Could you check a few things on this model? Use its own coordinates, in mm. Face numbers are marked on the shaded views. A direction names the side the tool comes from. Coordinates: 2 decimals unless noted, no trailing zeros. Write each loop counter-clockwise with the first axis right and the second up, starting at its lowest first coordinate (ties: lowest second). Pieces come first, ordered by that corner, then holes. Notation, with made-up numbers: (9, -24) - (19, -24) arc R23 ccw to (19, -9) - close; hole circle Ø10 at (-14, 58.5). An arc over 180 degrees is marked (long way). Answer as a JSON object with one key per item and string values. Group by question number.
1) On a 3-axis mill with a long thin cutter (end or side, diameter ignored), from which of +Z, -Z, +X, -X, +Y, -Y can I reach the whole of each face in a straight line? I mean the marked faces 1 and 2. Say none if no direction works.
2) If we section it at D-D (x = -20): Write out the boundary of the cut face in (y, z).
3) We'd pull the mould along Z, two halves only. Please class the marked faces 3 and 4: released by +Z, released by -Z, zero draft, split by the parting line, or undercut.
4) Will these pins go through, and if not, where does the flat tip stop? pin 1 Ø1 at (x, z) = (1.5, 21.5) entering from +Y; pin 2 Ø2 at (x, y) = (28, 6) entering from -Z; pin 3 Ø2 at (x, y) = (-30.5, 7) entering from +Z.
5) If we section it at B-B (z = 48): Write out the boundary of the cut face in (x, y).
6) Please list where these lines run through material, in increasing order: line 1 along Z through (x, y) = (-27.5, 5.5); line 2 along X through (y, z) = (20, 34.5); line 3 along Y through (x, z) = (-30, 4).
7) If we section it at C-C (y = 6.5): State how many separate pieces and enclosed holes the cut face has, plus the area to 3 significant figures.
8) If we section it at A-A (x = -30): Write out the boundary of the cut face in (y, z).
```python
from build123d import *

# Parameters (mm, degrees)
SKETCH1_W                                           = 75
SKETCH1_H                                           = 5
SKETCH1_W_2                                         = 5
SKETCH1_H_2                                         = 40
BOSS_EXTRUDE1_DEPTH                                 = 90
SKETCH2_R                                           = 2.1
CUT_EXTRUDE1_DEPTH                                  = 122.680935236
SKETCH4_W                                           = 4
SKETCH4_H                                           = 90
BOSS_EXTRUDE2_DEPTH                                 = 40
SKETCH6_W                                           = 7
SKETCH6_H                                           = 4
BOSS_EXTRUDE4_DEPTH                                 = 8
SKETCH7_R                                           = 1.6
CUT_EXTRUDE3_DEPTH                                  = 106.386194542
CUT_EXTRUDE4_REACH                                  = 126.624
LPATTERN1_COUNT                                     = 5
LPATTERN1_PITCH                                     = 12
SKETCH9_R                                           = 1.5
CUT_EXTRUDE5_DEPTH                                  = 104.834002138
CSK_FOR_M4_COUNTERSUNK_FLAT_HEAD_SCREW1_D           = 4
CSK_FOR_M4_COUNTERSUNK_FLAT_HEAD_SCREW1_CSINK_D     = 7.5
CSK_FOR_M4_COUNTERSUNK_FLAT_HEAD_SCREW1_CSINK_ANGLE = 90


with BuildPart() as part:
    # Sketch1 → Boss-Extrude1 (new body)
    with BuildSketch(Plane.XY):
        Rectangle(SKETCH1_W, SKETCH1_H)
        with Locations((35, 22.5)):
            Rectangle(SKETCH1_W_2, SKETCH1_H_2)
    extrude(amount=BOSS_EXTRUDE1_DEPTH)

    # Sketch2 → Cut-Extrude1 (cut, through all)
    with BuildSketch(Plane.ZY.offset(-32.5)):
        with Locations((20, 19.5)):
            Circle(SKETCH2_R)
        with Locations((70, 19.5)):
            Circle(SKETCH2_R)
    extrude(amount=-CUT_EXTRUDE1_DEPTH, mode=Mode.SUBTRACT)

    # Sketch4 → Boss-Extrude2 (add)
    with BuildSketch(Plane(origin=(0, 2.5, 0), x_dir=(1, 0, 0), z_dir=(0, 1, 0))):
        with Locations((-35.5, -45)):
            Rectangle(SKETCH4_W, SKETCH4_H)
    extrude(amount=BOSS_EXTRUDE2_DEPTH)

    # Sketch6 → Boss-Extrude4 (add)
    with BuildSketch(Plane(origin=(0, 2.5, 0), x_dir=(1, 0, 0), z_dir=(0, 1, 0))):
        with Locations((-30, -5)):
            Rectangle(SKETCH6_W, SKETCH6_H)
        with Locations((29, -5)):
            Rectangle(SKETCH6_W, SKETCH6_H)
        with Locations((29, -85)):
            Rectangle(SKETCH6_W, SKETCH6_H)
        with Locations((-30, -85)):
            Rectangle(SKETCH6_W, SKETCH6_H)
    extrude(amount=BOSS_EXTRUDE4_DEPTH)

    # Sketch7 → Cut-Extrude3 (cut, through all)
    with BuildSketch(Plane(origin=(0, 2.5, 0), x_dir=(1, 0, 0), z_dir=(0, 1, 0))):
        with Locations(Location((24.5, -68, 0), (0, 0, 180))):
            Circle(SKETCH7_R)
        with Locations(Location((-8.5, -17, 0), (0, 0, 180))):
            Circle(SKETCH7_R)
    extrude(amount=-CUT_EXTRUDE3_DEPTH, mode=Mode.SUBTRACT)

    # Sketch8 → Cut-Extrude4 (cut, up to next)
    with BuildSketch(Plane.ZY.offset(37.5), mode=Mode.PRIVATE) as cut_extrude4_sk1:
        with BuildLine():
            Line((32.061260163, 34.989949494), (32.202681519, 34.848528137))
            ThreePointArc((32.202681519, 34.848528137), (32.612732026, 33.858578644), (32.202681519, 32.86862915))
            Line((32.202681519, 32.86862915), (10.989949494, 11.655897124))
            ThreePointArc((10.989949494, 11.655897124), (10, 11.245846618), (9.010050506, 11.655897124))
            Line((9.010050506, 11.655897124), (8.86862915, 11.797318481))
            ThreePointArc((8.86862915, 11.797318481), (8.458578644, 12.787267974), (8.86862915, 13.777217468))
            Line((8.86862915, 13.777217468), (30.081361176, 34.989949494))
            ThreePointArc((30.081361176, 34.989949494), (31.07131067, 35.4), (32.061260163, 34.989949494))
        make_face()
    cut_extrude4_tool1 = extrude(cut_extrude4_sk1.sketch, amount=-CUT_EXTRUDE4_REACH, mode=Mode.PRIVATE) & part.part
    cut_extrude4 = cut_extrude4_tool1.solids().sort_by_distance((-37.5, 23.322923, 20.535655))[0]
    add(cut_extrude4, mode=Mode.SUBTRACT)

    # LPattern1: Cut-Extrude4 ×5
    with Locations(*[(0, 0, i * LPATTERN1_PITCH) for i in range(1, LPATTERN1_COUNT)]):
        add(cut_extrude4, mode=Mode.SUBTRACT)

    # Sketch9 → Cut-Extrude5 (cut, through all)
    with BuildSketch(Plane.XY.offset(87)):
        with Locations((-30, 6.5)):
            Circle(SKETCH9_R)
        with Locations((29, 6.5)):
            Circle(SKETCH9_R)
    extrude(amount=-CUT_EXTRUDE5_DEPTH, mode=Mode.SUBTRACT)

    # CSK for M4 Countersunk Flat Head Screw1 (through all)
    with Locations(Plane(origin=(24.5, -2.5, 68), x_dir=(0, 0, -1), z_dir=(0, -1, 0))):
        with Locations((0, 0), (51, -33)):
            CounterSinkHole(CSK_FOR_M4_COUNTERSUNK_FLAT_HEAD_SCREW1_D / 2, CSK_FOR_M4_COUNTERSUNK_FLAT_HEAD_SCREW1_CSINK_D / 2, counter_sink_angle=CSK_FOR_M4_COUNTERSUNK_FLAT_HEAD_SCREW1_CSINK_ANGLE)


solid = part.part
```
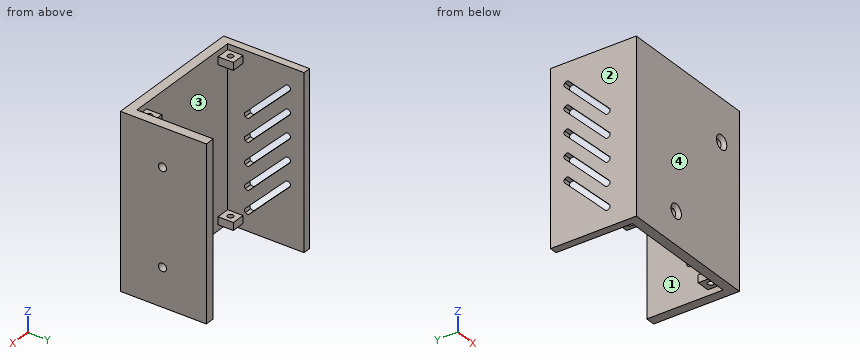
Here are the results:
{
 "1": {"face 1": "+Y", "face 2": "+Z, -Z, -X, +Y, -Y"},
 "2": {"outline": "(-2.5, 0) - (2.5, 0) - (2.5, 90) - (-2.5, 90) - close"},
 "3": {"face 3": "undercut", "face 4": "zero draft"},
 "4": {"pin 1": "stops at y = 2.5", "pin 2": "stops at z = 3", "pin 3": "stops at z = 87"},
 "5": {"outline": "(-37.5, -2.5) - (37.5, -2.5) - (37.5, 42.5) - (32.5, 42.5) - (32.5, 2.5) - (-33.5, 2.5) - (-33.5, 12.67) - (-37.5, 12.67) - close; (-37.5, 16.91) - (-33.5, 16.91) - (-33.5, 24.67) - (-37.5, 24.67) - close; (-37.5, 28.91) - (-33.5, 28.91) - (-33.5, 42.5) - (-37.5, 42.5) - close"},
 "6": {"line 1": "z = 3 to 7, 83 to 87", "line 2": "x = -37.5 to -33.5, 32.5 to 37.5", "line 3": "y = -2.5 to 5, 8 to 10.5"},
 "7": {"separate pieces": "6", "enclosed holes": "0", "area": "874 mm²"},
 "8": {"outline": "(-2.5, 0) - (2.5, 0) - (2.5, 3) - (5, 3) - (5, 7) - (2.5, 7) - (2.5, 83) - (5, 83) - (5, 87) - (2.5, 87) - (2.5, 90) - (-2.5, 90) - close; (8, 3) - (10.5, 3) - (10.5, 7) - (8, 7) - close; (8, 83) - (10.5, 83) - (10.5, 87) - (8, 87) - close"}
}
